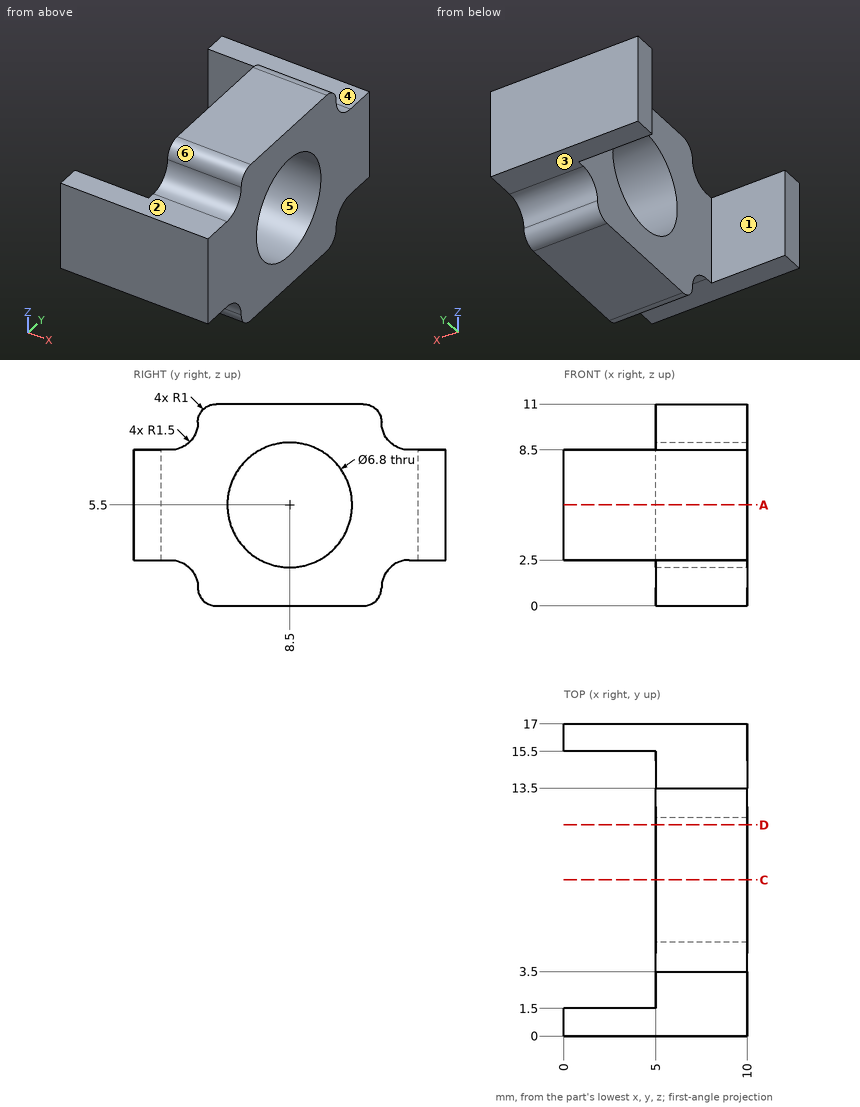
Could you check a few things on this drawing? It's one solid part, dimensions in mm from its lowest x, y, z. A direction names the side the tool comes from. Give positions to 0.01 mm unless a question says otherwise; leave off trailing zeros. Order: outer loops, then holes, each group sorted by start corner. A loop starts at its lowest first (then second) coordinate and runs counter-clockwise, first axis right, second up. Notation, with made-up numbers: M 77,71.5 L 92,71.5 A32 ccw 92,108.5 Z; hole C -9.5,85 d7. An arc over 180 degrees is marked long. Use one line per item in the form item = value. Start each with the question number.
Item 1: If we section it at A-A (z = 5.5): Write out the boundary of the cut face in (x, y), then the cut area to 3 significant figures.
Item 2: If we section it at C-C (y = 8.5): Write out the boundary of the cut face in (x, z).
Item 3: If we section it at D-D (y = 11.5): Write out the boundary of the cut face in (x, z).
Item 4: For the marked faces 1, 2 and 3, which set-ups out of +Z, -Z, +X, -X, +Y, -Y let a thin tool reach every point of the face, with its end or its side?
Item 5: If I drill on line 1 along Y through (x, z) = (8.4, 5.5); line 2 along Y through (x, z) = (1.5, 8.25); line 3 along X through (y, z) = (3.75, 4.5), over which ranges is the centre line in solid material (lowest first)?
Item 6: Will these pins go through, and if not, where does the flat tip stop? pin 1 Ø2 at (x, y) = (4.5, 0.5) entering from +Z; pin 2 Ø1 at (x, y) = (3, 1) entering from -Z.
Item 7: We'd pull the mould along Y, two halves only. Please class the marked faces 4, 5 and 6: +Y half, -Y half, draft (parallel to the pull), parting line (faces both ways), or undercut.
Outcome:
q1.outline = M 0,0 L 10,0 L 10,5.1 L 5,5.1 L 5,1.5 L 0,1.5 Z; M 0,15.5 L 5,15.5 L 5,11.9 L 10,11.9 L 10,17 L 0,17 Z
q1.area = 66.0 mm2
q2.outline = M 5,0 L 10,0 L 10,2.1 L 5,2.1 Z; M 5,8.9 L 10,8.9 L 10,11 L 5,11 Z
q3.outline = M 5,0 L 10,0 L 10,3.9 L 5,3.9 Z; M 5,7.1 L 10,7.1 L 10,11 L 5,11 Z
q4.face_1 = +Z, -Z, -X
q4.face_2 = +Z, +X, -X, -Y
q4.face_3 = -Z, +X, -X, +Y
q5.line_1 = 0 to 5.1, 11.9 to 17
q5.line_2 = 0 to 1.5, 15.5 to 17
q5.line_3 = 5 to 10
q6.pin_1 = 8.5
q6.pin_2 = 2.5
q7.face_4 = draft
q7.face_5 = undercut
q7.face_6 = -Y half
